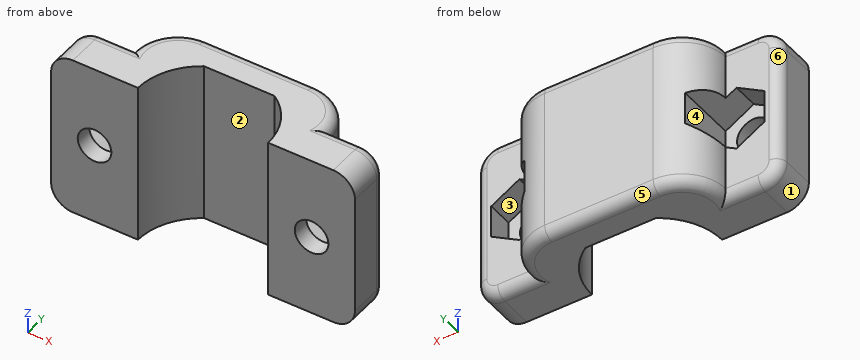
Autodesk Inventor part; units mm, degrees
ref_plane "Work Plane1" through (2.4271, -3.6326, 0) normal (-1, 0, 0) x (0, 0, 1)
ref_plane "Work Plane2" through (0, 0, 7.5) normal (0, 0, 1) x (1, 0, 0)
ref_plane "YZ Plane" through (0, 0, 0) normal (1, 0, 0) x (0, 1, 0)
sketch "Sketch3" plane through (0, 0, 0) normal (0, 0, 1) x (1, 0, 0)
  line L0 (2.4271, 1.3674) -> (5.6771, 1.3674)
  arc A0 (8.4273, -3.6326) -> (5.6771, 1.3674) centre (2.5072, -3.6326) ccw
  line L1 (8.4273, -3.6326) -> (8.4273, -3.6326)
  line L2 (8.4273, -3.6326) -> (16.4273, -3.6326)
  line L3 (16.4273, -3.6326) -> (16.4273, 0.3674)
  line L4 (16.4273, 0.3674) -> (11.4273, 0.3674)
  line L5 (2.4271, 4.3674) -> (7.4273, 4.3674)
  line L6 (11.4273, 0.3674) -> (11.4273, 0.3674)
  arc A1 (11.4273, 0.3674) -> (7.4273, 4.3674) centre (7.4273, 0.3674) ccw
  arc A2 (-0.8229, 1.3674) -> (-3.5732, -3.6326) centre (2.3469, -3.6326) ccw
  line L7 (-3.5732, -3.6326) -> (-3.5732, -3.6326)
  line L8 (-3.5732, -3.6326) -> (-11.5732, -3.6326)
  line L9 (-11.5732, -3.6326) -> (-11.5732, 0.3674)
  line L10 (-11.5732, 0.3674) -> (-6.5732, 0.3674)
  line L11 (-6.5732, 0.3674) -> (-6.5732, 0.3674)
  arc A3 (-2.5732, 4.3674) -> (-6.5732, 0.3674) centre (-2.5732, 0.3674) ccw
  line L12 (2.4271, 4.3674) -> (-2.5732, 4.3674)
  line L13 (2.4271, 1.3674) -> (-0.8229, 1.3674)
  point P0 (0, 0)
  point P1 (11.4273, 0.3674)
  point P2 (-6.5732, 0.3674)
  dimension "d20" = 4
  dimension "d21" = 5
  dimension "d22" = 8
  dimension "d23" = 3
extrude "Extrusion2" add sketch "Sketch3" along normal blind 15
ref_plane "Work Plane1" through (2.4271, -3.6326, 0) normal (-1, 0, 0) x (0, 0, 1)
sketch "Sketch4" plane through (-11.5732, 0.3674, 0) normal (0, 1, 0) x (1, 0, 0)
  line L0 (4, -4.495) -> (6.6024, -5.9975)
  line L1 (6.6024, -5.9975) -> (6.6024, -9.0025)
  line L2 (6.6024, -9.0025) -> (4, -10.505)
  line L3 (4, -10.505) -> (1.3976, -9.0025)
  line L4 (1.3976, -9.0025) -> (1.3976, -5.9975)
  line L5 (1.3976, -5.9975) -> (4, -4.495)
  line L6 (0, 0) -> (0, -15)
  line L7 (14.0003, -18) -> (14.0003, 3)
  line L8 (5, 0) -> (0, 0)
  point P0 (11.5732, 0)
  point P1 (4, -7.5)
  point P2 (4, -7.5)
  dimension "d26" = 6.01
  dimension "d27" = 4
  dimension "d39" = 7.5
extrude "Extrusion3" cut sketch "Sketch4" along normal blind 8 and the other way blind 2.4
sketch "Sketch5" plane through (-11.5732, -2.0326, 0) normal (0, 1, 0) x (1, 0, 0)
  line L0 (6.6024, -5.9975) -> (6.6024, -9.0025)
  line L1 (1.3976, -9.0025) -> (1.3976, -5.9975)
  line L2 (5, 0) -> (0, 0)
  point P0 (11.5732, 0)
  point P1 (4, -7.5)
  dimension "d40" = 7.5
hole "Hole1" at (-7.5732, -2.0326, 7.5) direction (0, -1, 0) diameter 3.1 end through all
mirror "Mirror1" about plane through (2.4271, -3.6326, 0) normal (-1, 0, 0) of "Extrusion3", "Hole1"
ref_plane "Work Plane2" through (0, 0, 7.5) normal (0, 0, 1) x (1, 0, 0)
fillet "Fillet3" radius 2 4 edges at (16.4273, -1.6326, 0) (16.4273, -1.6326, 15) (-11.5732, -1.6326, 15) (-11.5732, -1.6326, 0)
fillet "Fillet4" radius 1 16 edges at (15.8415, 0.3674, 0.5858) (16.4273, 0.3674, 7.5) (15.8415, 0.3674, 14.4142) (12.9273, 0.3674, 15) (12.9273, 0.3674, 0) (2.4271, 4.3674, 0) (-5.4016, 3.1958, 0) (10.2558, 3.1958, 0) (-8.0732, 0.3674, 0) (-11.5732, 0.3674, 7.5) (-10.9874, 0.3674, 14.4142) (-8.0732, 0.3674, 15) (-10.9874, 0.3674, 0.5858) (2.4271, 4.3674, 15) (10.2558, 3.1958, 15) (-5.4016, 3.1958, 15)
properties part number "mocowanie_silnika_CPY" material "ABS Plastic"
Work out the finished part from the listing and answer in its coordinate system (mm). Face numbers are marked on the shaded views. A direction names the side the tool comes from. Round coordinates to 2 decimals unless told otherwise and drop trailing zeros. Order: outer loops, then holes, each group sorted by start corner. A loop starts at its lowest first (then second) coordinate and runs counter-clockwise, first axis right, second up. Notation, with made-up numbers: M 10.25,-28.75 L 51.25,-28.75 A14 cw 51.25,-1.75 Z; hole C -18,9.25 d11. An arc over 180 degrees is marked long. One line per item, written item: value.
Q1. Determine the mould class of the marked faces 4, 5 and 6 for opening direction X: released by +X, released by -X, zero draft, split by the parting line, or undercut.
Derived:
face 4: undercut
face 5: zero draft
face 6: released by -X
Q2. For the marked faces 1, 2 and 3, determine the directions among +Z, -Z, +X, -X, +Y, -Y from which every point of the face is accessible in a straight line to the end or side of a thin tool.
Derived:
face 1: -Z, -X, +Y, -Y
face 2: +Z, -Z, -Y
face 3: +Y
Q3. Find section C-C on x = 2.5. Write down the section's boundary in (y, z), then the cut area to 3 significant figures.
Derived:
outline: M 1.37,0 L 3.37,0 A1 ccw 4.37,1 L 4.37,14 A1 ccw 3.37,15 L 1.37,15 Z
area: 44.6 mm²
Q4. Flat-ended cylindrical pins translate along their axes: pin 1 (4.5 mm diameter, centred on x = -9.5, z = 8, fed in from +Y); pin 2 (5 mm diameter, centred on x = 3, z = 4.5, fed in from -Y); pin 3 (2.5 mm diameter, centred on y = 2, z = 7.5, fed in from +X) (3 decimals). Find the tip coordinate at first contact, or state that the pin passes through.
Derived:
pin 1: y = 0.37
pin 2: y = 1.37
pin 3: x = 9.825
Q5. Find section B-B on z = 7.5. Write down the section's boundary in (x, y) (3 decimals).
Derived:
outline: M -11.573,-3.633 L -9.123,-3.633 L -9.123,-2.033 L -10.176,-2.033 L -10.176,0.367 L -10.573,0.367 A1 ccw -11.573,-0.633 Z; M -6.023,-3.633 L -3.573,-3.633 A5.92 cw -0.823,1.367 L 5.677,1.367 A5.92 cw 8.427,-3.633 L 10.877,-3.633 L 10.877,-2.033 L 9.825,-2.033 L 9.825,3.569 A4 ccw 7.427,4.367 L -2.573,4.367 A4 ccw -4.971,3.569 L -4.971,-2.033 L -6.023,-2.033 Z; M 13.977,-3.633 L 16.427,-3.633 L 16.427,-0.633 A1 ccw 15.427,0.367 L 15.03,0.367 L 15.03,-2.033 L 13.977,-2.033 Z
Q6. Find section A-A on z = 3. Write down the section's boundary in (x, y).
Derived:
outline: M -11.57,-3.63 L -3.57,-3.63 A5.92 cw -0.82,1.37 L 5.68,1.37 A5.92 cw 8.43,-3.63 L 16.43,-3.63 L 16.43,-0.63 A1 ccw 15.43,0.37 L 11.43,0.37 A4 ccw 7.43,4.37 L -2.57,4.37 A4 ccw -6.57,0.37 L -10.57,0.37 A1 ccw -11.57,-0.63 Z
Q7. Straight lines are drawn through the part: line 1 (X direction, y = -2.5, z = 7.5); line 2 (X direction, y = -3.05, z = 7.5); line 3 (Y direction, x = 3.5, z = 1.5). For each, find the intervals that lie inside material, in ascending order.
Derived:
line 1: -11.57 to -9.12, -6.02 to -3.46, 8.32 to 10.88, 13.98 to 16.43
line 2: -11.57 to -9.12, -6.02 to -3.54, 8.4 to 10.88, 13.98 to 16.43
line 3: 1.37 to 4.37
